Here's how the part is built. I have some questions about the finished solid (model axes, mm). Face numbers are marked on the shaded views. A direction names the side the tool comes from. Coordinates: 2 decimals unless noted, no trailing zeros. Loops run counter-clockwise (first coordinate to the right, second up) from the corner with the lowest first, then second, coordinate; pieces in that order, holes last. Notation, with made-up numbers: M -7.5,51 L 2.5,51 A13 ccw 2.5,63 Z; hole C 62.5,-28 d6. An arc over 180 degrees is marked long. Use one line per item in the form item = value. Start each with the question number.
(1) Imagine slicing it at A-A, the plane z = 2. Please give me the cut outline in (x, y), and give its area (3 significant figures).
(2) Imagine slicing it at B-B, the plane y = -7.55. Please give me the cut outline in (x, z), and give its area (3 significant figures).
(3) Imagine slicing it at D-D, the plane x = -0.75. Please give me the cut outline in (y, z).
(4) On a 3-axis mill with a long thin cutter (end or side, diameter ignored), from which of +Z, -Z, +X, -X, +Y, -Y can I reach the whole of each face in a straight line? I mean the marked faces 1, 2 and 3. Say none if no direction works.
(5) Will these pins go through, and if not, where does the flat tip stop? P1, Ø3.5, axis at x = -7, z = 5, coming from the +Y side; P2, Ø1.7, axis at x = -5, y = -5.5, coming from the +Z side; P3, Ø4, axis at x = -0.5, z = -12, coming from the +Y side; P4, Ø0.6, axis at x = 10, y = -3, coming from the -Z side.
(6) Imagine slicing it at C-C, the plane z = -23. Please give me the cut outline in (x, y).
(7) Please list where these lines run through material, in increasing order: L1, parallel to Z at x = 1, y = -7.95; L2, parallel to Z at x = 6.5, y = -5.35; L3, parallel to Z at x = 7.5, y = -6.2.
(8) Thinking about a two-plate mould opening in Z: for the marked faces 4, 5, 6 and 7, which applies, +Z half, -Z half, draft (parallel to the pull), parting line (faces both ways), or undercut?
```python
from build123d import *

# Parameters (mm, degrees)
SKETCH1_W           = 20.6
SKETCH1_H           = 17.2
BOSS_EXTRUDE1_DEPTH = 2.5
SKETCH2_W           = 20.6
SKETCH2_H           = 1.5
BOSS_EXTRUDE2_DEPTH = 25.3
SKETCH3_W           = 20.6
SKETCH3_H           = 5
BOSS_EXTRUDE3_DEPTH = 1
SKETCH4_W           = 3.35
SKETCH4_H           = 25.3
BOSS_EXTRUDE4_DEPTH = 4
CUT_EXTRUDE2_START  = 25.3
CUT_EXTRUDE2_DEPTH  = 25.3
CHAMFER1_SIZE       = 2
BOSS_EXTRUDE5_DEPTH = 1.2
SKETCH7_W           = 4.5
SKETCH7_H           = 5
BOSS_EXTRUDE6_DEPTH = 1.5
SKETCH8_R           = 16.793205084
CUT_EXTRUDE3_DEPTH  = 2.5
BOSS_EXTRUDE7_DEPTH = 11.1
BOSS_EXTRUDE8_DEPTH = 1
SKETCH11_W          = 4.5
SKETCH11_H          = 5
BOSS_EXTRUDE9_DEPTH = 2
CHAMFER2_SIZE       = 2
SKETCH12_W          = 13.9
SKETCH12_H          = 24.3
CUT_EXTRUDE4_DEPTH  = 1


with BuildPart() as part:
    # Sketch1 → Boss-Extrude1 (new body)
    with BuildSketch(Plane.XY):
        Rectangle(SKETCH1_W, SKETCH1_H)
        with BuildLine():
            Line((3.1, 2.3), (3.1, -2))
            ThreePointArc((3.1, -2), (0, -5.1), (-3.1, -2))
            Line((-3.1, -2), (-3.1, 2.3))
            ThreePointArc((-3.1, 2.3), (0, 5.4), (3.1, 2.3))
        make_face(mode=Mode.SUBTRACT)
    extrude(amount=BOSS_EXTRUDE1_DEPTH)

    # Sketch2 → Boss-Extrude2 (add)
    with BuildSketch(Plane(origin=(0, 0, 0), x_dir=(-1, 0, 0), z_dir=(0, 0, -1))):
        with Locations((0, -7.85)):
            Rectangle(SKETCH2_W, SKETCH2_H)
    extrude(amount=BOSS_EXTRUDE2_DEPTH)

    # Sketch3 → Boss-Extrude3 (add)
    with BuildSketch(Plane(origin=(0, 0, -25.3), x_dir=(-1, 0, 0), z_dir=(0, 0, -1))):
        with Locations((0, -6.1)):
            Rectangle(SKETCH3_W, SKETCH3_H)
    extrude(amount=BOSS_EXTRUDE3_DEPTH)

    # Sketch4 → Boss-Extrude4 (add)
    with BuildSketch(Plane(origin=(0, -7.1, 0), x_dir=(1, 0, 0), z_dir=(0, 1, 0))):
        with Locations((-8.625, 12.65)):
            Rectangle(SKETCH4_W, SKETCH4_H)
        with Locations((8.625, 12.65)):
            Rectangle(SKETCH4_W, SKETCH4_H)
    extrude(amount=BOSS_EXTRUDE4_DEPTH)

    # Sketch5 → Cut-Extrude2 (cut)
    # profile 1 of 3: a face of its own
    with BuildSketch(Plane(origin=(0, 0, 0), x_dir=(-1, 0, 0), z_dir=(0, 0, -1)).offset(CUT_EXTRUDE2_START)):
        with BuildLine():
            Line((-6.800183821, -7.1), (6.800183821, -7.1))
            ThreePointArc((6.800183821, -7.1), (6.87545093, -7.030121044), (6.95, -6.959476565))
            Line((6.95, -6.959476565), (6.95, -3.1))
            Line((6.95, -3.1), (9.457404507, -3.1))
            ThreePointArc((9.457404507, -3.1), (9.900742783, -1.425628104), (10.05, 0.3))
            ThreePointArc((10.05, 0.3), (8.886892922, 4.993147579), (5.666789214, 8.6))
            Line((5.666789214, 8.6), (-5.666789214, 8.6))
            ThreePointArc((-5.666789214, 8.6), (-9.560743116, 3.397529834), (-9.457404507, -3.1))
            Line((-9.457404507, -3.1), (-6.95, -3.1))
            Line((-6.95, -3.1), (-6.95, -6.959476565))
            ThreePointArc((-6.95, -6.959476565), (-6.87545093, -7.030121044), (-6.800183821, -7.1))
        make_face()
        with BuildLine():
            ThreePointArc((3.1, -2), (0, -5.1), (-3.1, -2))
            Line((-3.1, -2), (-3.1, 2.3))
            ThreePointArc((-3.1, 2.3), (0, 5.4), (3.1, 2.3))
            Line((3.1, 2.3), (3.1, -2))
        make_face(mode=Mode.SUBTRACT)
    # profile 2 of 3: a face of its own
    with BuildSketch(Plane(origin=(0, 0, 0), x_dir=(-1, 0, 0), z_dir=(0, 0, -1)).offset(CUT_EXTRUDE2_START)):
        with BuildLine():
            Line((6.95, -3.1), (6.95, -6.959476565))
            ThreePointArc((6.95, -6.959476565), (8.427610604, -5.175205887), (9.457404507, -3.1))
            Line((9.457404507, -3.1), (6.95, -3.1))
        make_face()
    # profile 3 of 3: a face of its own
    with BuildSketch(Plane(origin=(0, 0, 0), x_dir=(-1, 0, 0), z_dir=(0, 0, -1)).offset(CUT_EXTRUDE2_START)):
        with BuildLine():
            ThreePointArc((-9.457404507, -3.1), (-8.427610604, -5.175205887), (-6.95, -6.959476565))
            Line((-6.95, -6.959476565), (-6.95, -3.1))
            Line((-6.95, -3.1), (-9.457404507, -3.1))
        make_face()
    extrude(amount=-CUT_EXTRUDE2_DEPTH, mode=Mode.SUBTRACT)

    # Chamfer1
    chamfer1_edges = [part.edges().sort_by_distance(p)[0] for p in [
        (-10.3, 8.6, 1.25),
        (10.3, 8.6, 1.25),
    ]]
    chamfer(chamfer1_edges, length=CHAMFER1_SIZE)

    # Sketch6 → Boss-Extrude5 (add)
    with BuildSketch(Plane(origin=(0, 0, -26.3), x_dir=(-1, 0, 0), z_dir=(0, 0, -1))):
        Polygon((-7.3, -8.6), (-10.3, -8.6), (-10.3, -3.6), (-9.3, -3.6), align=None)
        Polygon((9.3, -3.6), (7.3, -8.6), (10.3, -8.6), (10.3, -3.6), align=None)
    extrude(amount=BOSS_EXTRUDE5_DEPTH)

    # Sketch7 → Boss-Extrude6 (add)
    with BuildSketch(Plane(origin=(0, 0, -27.5), x_dir=(-1, 0, 0), z_dir=(0, 0, -1))):
        with Locations((-8.05, -6.1)):
            Rectangle(SKETCH7_W, SKETCH7_H)
        with Locations((8.05, -6.1)):
            Rectangle(SKETCH7_W, SKETCH7_H)
    extrude(amount=-BOSS_EXTRUDE6_DEPTH)

    # Sketch8 → Cut-Extrude3 (cut)
    with BuildSketch(Plane.XY.offset(2.5)):
        Circle(SKETCH8_R)
    extrude(amount=-CUT_EXTRUDE3_DEPTH, mode=Mode.SUBTRACT)

    # Sketch9 → Boss-Extrude7 (add)
    with BuildSketch(Plane.XY):
        Polygon((7.3, -8.6), (10.3, -8.6), (10.3, -3.6), (9.3, -3.6), align=None)
        Polygon((-10.3, -8.6), (-7.3, -8.6), (-9.3, -3.6), (-10.3, -3.6), align=None)
    extrude(amount=BOSS_EXTRUDE7_DEPTH)

    # Sketch10 → Boss-Extrude8 (add)
    with BuildSketch(Plane.XY.offset(2.6)):
        Polygon((-9.3, -3.6), (-7.3, -3.6), (-7.3, -8.6), (-10.3, -8.6), (-10.3, -3.6), align=None)
        Polygon((9.3, -3.6), (7.3, -3.6), (7.3, -8.6), (10.3, -8.6), (10.3, -3.6), align=None)
    extrude(amount=BOSS_EXTRUDE8_DEPTH)

    # Sketch11 → Boss-Extrude9 (add)
    with BuildSketch(Plane.XY.offset(11.1)):
        with Locations((-8.05, -6.1)):
            Rectangle(SKETCH11_W, SKETCH11_H)
        with Locations((8.05, -6.1)):
            Rectangle(SKETCH11_W, SKETCH11_H)
    extrude(amount=-BOSS_EXTRUDE9_DEPTH)

    # Chamfer2
    chamfer2_edges = [part.edges().sort_by_distance(p)[0] for p in [
        (5.8, -3.6, 10.1),
    ]]
    chamfer(chamfer2_edges, length=CHAMFER2_SIZE)

    # Sketch12 → Cut-Extrude4 (cut)
    with BuildSketch(Plane(origin=(0, -7.1, 0), x_dir=(1, 0, 0), z_dir=(0, 1, 0))):
        with Locations((0, 13.15)):
            Rectangle(SKETCH12_W, SKETCH12_H)
    extrude(amount=-CUT_EXTRUDE4_DEPTH, mode=Mode.SUBTRACT)


solid = part.part
```
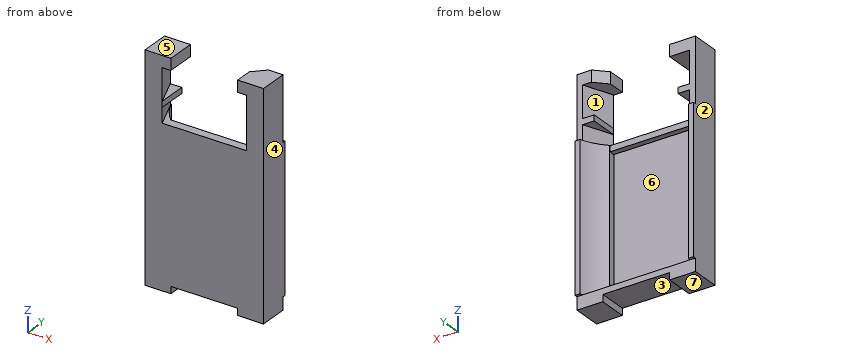
Answer:
q1.outline = M -10.3,-8.6 L -7.3,-8.6 L -9.3,-3.6 L -10.3,-3.6 Z; M 7.3,-8.6 L 10.3,-8.6 L 10.3,-3.6 L 9.3,-3.6 Z
q1.area = 20.0 mm²
q2.outline = M -10.3,-27.5 L -5.8,-27.5 L -5.8,-26.3 L 5.8,-26.3 L 5.8,-27.5 L 10.3,-27.5 L 10.3,11.1 L 5.8,11.1 L 5.8,9.1 L 7.72,9.1 L 7.72,3.6 L 7.3,3.6 L 7.3,2.6 L 7.72,2.6 L 7.72,0 L -7.72,0 L -7.72,2.6 L -7.3,2.6 L -7.3,3.6 L -7.72,3.6 L -7.72,9.1 L -5.8,9.1 L -5.8,11.1 L -10.3,11.1 Z; hole M -6.95,-25.3 L 6.95,-25.3 L 6.95,-1 L -6.95,-1 Z
q2.area = 281 mm²
q3.outline = M -8.6,-26.3 L -3.6,-26.3 L -3.6,-25.3 L -8.1,-25.3 L -8.1,-1 L -7.1,-1 L -7.1,0 L -8.6,0 Z
q4.face_1 = +Y
q4.face_2 = +Z, -Z, -X, +Y, -Y
q4.face_3 = -Z, +Y, -Y
q5.P1 = -3.6
q5.P2 = 11.1
q5.P3 = -8.1
q5.P4 = -25.3
q6.outline = M -10.3,-8.6 L 10.3,-8.6 L 10.3,-3.1 L 9.46,-3.1 A10.05 cw 6.95,-6.96 L 6.95,-8.1 L -6.95,-8.1 L -6.95,-6.96 A10.05 cw -9.46,-3.1 L -10.3,-3.1 Z
q7.L1 = -26.3 to -25.3, -1 to 0
q7.L2 = -27.5 to -25.3, 9.1 to 11.1
q7.L3 = -27.5 to -25.3, 2.6 to 3.6, 9.1 to 11.1
q8.face_4 = draft
q8.face_5 = +Z half
q8.face_6 = undercut
q8.face_7 = -Z half
